```python
from build123d import *

# Parameters (mm, degrees)
SKETCH1_R                               = 20
BLOCO_DEPTH                             = 22
ENCAIXE_START                           = -18
ENCAIXE_DO_POTENCI_METRO_DEPTH          = 18
FURO_DE_FIXA_O_PARAFUSO_M3_D            = 3.6
FURO_DE_FIXA_O_PARAFUSO_M3_CBORE_D      = 6.5
FURO_DE_FIXA_O_PARAFUSO_M3_CBORE_DEPTH  = 3
CORTE_ARREDONDAMENTO_DEPTH              = 36.832945734
CORTE_ARREDONDAMENTO_DEPTH_BACK         = 36.832945734
SKETCH7_R                               = 100
SKETCH7_R_2                             = 75
FURO_DE_FIXA_O_POTENCI_METRO_REACH      = 37.833
FURO_DE_FIXA_O_POTENCI_METRO_END_RADIUS = 20
SKETCH8_R                               = 1.5


with BuildPart() as part:
    # Sketch1 → Bloco (new body)
    with BuildSketch(Plane(origin=(0, 0, 0), x_dir=(0, 0, -1), z_dir=(1, 0, 0))):
        Circle(SKETCH1_R)
    extrude(amount=BLOCO_DEPTH)

    # Sketch2 → Encaixe do Potenciômetro (cut)
    with BuildSketch(Plane(origin=(22, 0, 0), x_dir=(0, 0, -1), z_dir=(1, 0, 0)).offset(ENCAIXE_START)):
        with BuildLine():
            Line((-8, -18.33030278), (-8, -2.015564437))
            ThreePointArc((-8, -2.015564437), (0, 8.25), (8, -2.015564437))
            Line((8, -2.015564437), (8, -18.33030278))
            ThreePointArc((8, -18.33030278), (0, -20), (-8, -18.33030278))
        make_face()
    extrude(amount=ENCAIXE_DO_POTENCI_METRO_DEPTH, mode=Mode.SUBTRACT)

    # Furo de Fixação - Parafuso M3 (through all)
    with Locations(Plane.ZY):
        with Locations((10.606601718, 10.606601718), (-10.606601718, -10.606601718)):
            CounterBoreHole(FURO_DE_FIXA_O_PARAFUSO_M3_D / 2, FURO_DE_FIXA_O_PARAFUSO_M3_CBORE_D / 2, FURO_DE_FIXA_O_PARAFUSO_M3_CBORE_DEPTH)

    # Sketch7 → Corte - Arredondamento (cut, two sides: drawn at the far end of the back side and taken through both)
    with BuildSketch(Plane(origin=(0, 0, 0), x_dir=(1, 0, 0), z_dir=(0, 1, 0)).offset(-CORTE_ARREDONDAMENTO_DEPTH_BACK)):
        with Locations((75, 0)):
            Circle(SKETCH7_R)
        with Locations((75, 0)):
            Circle(SKETCH7_R_2, mode=Mode.SUBTRACT)
    extrude(amount=CORTE_ARREDONDAMENTO_DEPTH + CORTE_ARREDONDAMENTO_DEPTH_BACK, mode=Mode.SUBTRACT)

    # Furo de Fixação - Potenciômetro: up to this cylinder (the profile starts inside it)
    furo_de_fixa_o_potenci_metro_end = Plane(origin=(7, 0, 0), z_dir=(-1, 0, 0)) * Cylinder(FURO_DE_FIXA_O_POTENCI_METRO_END_RADIUS, 116.666, mode=Mode.PRIVATE)
    # Sketch8 → Furo de Fixação - Potenciômetro (cut, up to the surface)
    with BuildSketch(Plane.XY, mode=Mode.PRIVATE) as furo_de_fixa_o_potenci_metro_sk1:
        with Locations(Location((7, 0, 0), (0, 0, 180))):
            Circle(SKETCH8_R)
    furo_de_fixa_o_potenci_metro_tool1 = extrude(furo_de_fixa_o_potenci_metro_sk1.sketch, amount=FURO_DE_FIXA_O_POTENCI_METRO_REACH, mode=Mode.PRIVATE) & furo_de_fixa_o_potenci_metro_end
    add(furo_de_fixa_o_potenci_metro_tool1.solids().sort_by_distance((7, 0, 0))[0], mode=Mode.SUBTRACT)


solid = part.part
```
The model under review builds one solid part; all positions refer to its coordinate system, in mm. A direction names the side the tool comes from. Coordinates: 2 decimals unless noted, no trailing zeros. Write each loop counter-clockwise with the first axis right and the second up, starting at its lowest first coordinate (ties: lowest second). Pieces come first, ordered by that corner, then holes.
1) We need section C-C on z = 10. State the section outline as (x, y) points, then the cut area to 3 significant figures.
2) We need section A-A on x = 6.5. State the section outline as (y, z) points, then the cut area to 3 significant figures.
3) To check wall thickness, follow probe 1 along Y at (x, z) = (7, 10.5); probe 2 along Y at (x, z) = (18.5, -9.5); probe 3 along Z at (x, y) = (5.5, 2). State the ranges of each line that lie inside material, in increasing order.
4) Machinability: for faces 1 (the face through (12.874, 8.247, 0.21)), 2 (the face through (1.95, 10.75, 7.36)), 3 (the face through (13, -10, 8)), which of the approach directions +Z, -Z, +X, -X, +Y, -Y give a long, thin tool a straight path to every point of the face, cutting with its end or side? Answer none if there is none.
5) We need section D-D on z = -10.5. State the section outline as (x, y) points, then the cut area to 3 significant figures.
6) The part is to be moulded in two halves that separate along X. For faces 4 (the face through (13, -10, -8)), 5 (the face through (8.5, -0.07, 13.97)), 6 (the face through (22, 10, 0)), say which applies: pulls with the +X half, pulls with the -X half, needs draft (parallel to the pull), parting line crosses it, or undercut.
7) We need section B-B on y = 0. State the section outline as (x, z) points.
8) Clearance check with flat-ended pins moving along their axes: pin 1 Ø10.5 at (y, z) = (10.61, 10.61) entering from -X; pin 2 Ø3 at (x, z) = (4, -6) entering from -Y; pin 3 Ø10 at (y, z) = (0, 0) entering from +X. State where each tip first meets the part, or that it passes through.
Answer list:
1. outline: (0.67, -17.32) - (22, -17.32) - (22, 8.91) - (3, 8.91) - (3, 7.41) - (0.67, 7.41) - close; (0.67, 13.8) - (3, 13.8) - (3, 12.3) - (22, 12.3) - (22, 17.32) - (0.67, 17.32) - close; hole circle Ø3 at (7, 0)
1. area: 653 mm2
2. outline: (-18.33, -8) arc R20 ccw (long way) to (1.41, 19.95) - (1.41, 8.13) arc R8.25 cw (long way) to (-2.02, -8) - close; (-18.33, 8) - (-2.02, 8) arc R8.25 cw to (-1.41, 8.13) - (-1.41, 19.95) arc R20 ccw to start; hole circle Ø3.6 at (-10.61, -10.61); hole circle Ø3.6 at (10.61, 10.61)
2. area: 784 mm2
3. probe 1: y = -17.02 to -1.5, 1.5 to 8.81, 12.4 to 17.02
3. probe 2: y = -17.6 to -12.03, -9.19 to 17.6
3. probe 3: z = -19.9 to -8, 8 to 19.9
4. face 1: +X
4. face 2: -X
4. face 3: +X, -Y
5. outline: (0.74, -17.02) - (22, -17.02) - (22, -12.4) - (3, -12.4) - (3, -13.85) - (0.74, -13.85) - close; (0.74, -7.36) - (3, -7.36) - (3, -8.81) - (22, -8.81) - (22, 17.02) - (0.74, 17.02) - close
5. area: 641 mm2
6. face 4: needs draft
6. face 5: undercut
6. face 6: pulls with the +X half
7. outline: (2.72, -20) - (22, -20) - (22, -8.25) - (4, -8.25) - (4, 8.25) - (5.5, 8.25) - (5.5, 20) - (2.72, 20) arc R75 ccw to start; (8.5, 8.25) - (22, 8.25) - (22, 20) - (8.5, 20) - close
8. pin 1: stops at x = 0.19
8. pin 2: stops at y = -19.49
8. pin 3: stops at x = 4
